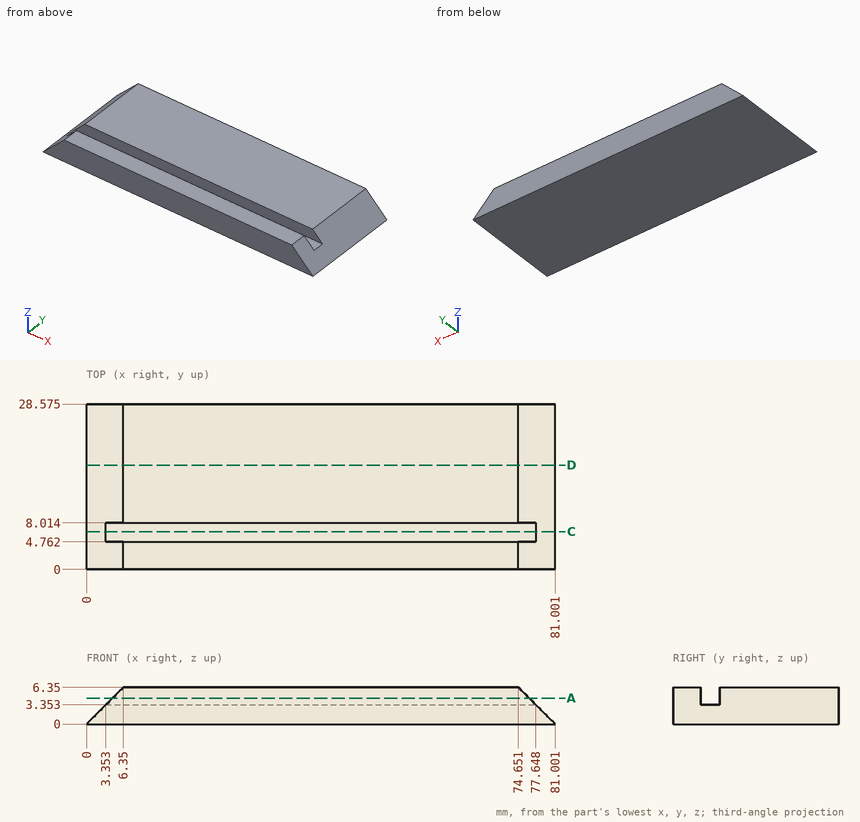
Study the drawing (mm; zero at the part's minimum x, y, z) and answer. Give positions to 0.01 mm unless a question says otherwise; leave off trailing zeros. Write each loop counter-clockwise with the first axis right and the second up, starting at its lowest first coordinate (ties: lowest second). Pieces come first, ordered by that corner, then holes. Notation, with made-up numbers: (-2.5, -23) -> (46.5, -23) arc R29 ccw to (46.5, -2) -> close; hole circle Ø4 at (34, 19.5). An arc over 180 degrees is marked (long way). Answer as a JSON object with one key per item and string values. Group by question number.
1) Find section D-D (y = 18). Write down the section's boundary in (x, z), and give its area (3 significant figures).
2) Find section A-A (z = 4.5). Write down the section's boundary in (x, y) (1 decimal), and give its area (3 significant figures).
3) Consider L1, parallel to Y at x = 24.5, z = 4 (1 decimal); L2, parallel to Z at x = 23.5, y = 5.25; L3, parallel to X at y = 23.25, z = 4. Determine where each line is inside the solid, lowest interval first. Write a range as from..to.
4) Find section C-C (y = 6.5). Write down the section's boundary in (x, z).
Values follow:
{
 "1": {"outline": "(0, 0) -> (81, 0) -> (74.65, 6.35) -> (6.35, 6.35) -> close", "area": "474 mm2"},
 "2": {"outline": "(4.5, 0) -> (76.5, 0) -> (76.5, 4.8) -> (4.5, 4.8) -> close; (4.5, 8) -> (76.5, 8) -> (76.5, 28.6) -> (4.5, 28.6) -> close", "area": "1,820 mm2"},
 "3": {"L1": "y = 0..4.8, 8..28.6", "L2": "z = 0..3.35", "L3": "x = 4..77"},
 "4": {"outline": "(0, 0) -> (81, 0) -> (77.65, 3.35) -> (3.35, 3.35) -> close"}
}
